```python
from build123d import *

# Parameters (mm, degrees)
EXTRUDE_1_DEPTH          = 3.5
EXTRUDE_1_DEPTH_BACK     = 3.5
SKETCH_1_R               = 2
EXTRUDE_2_DEPTH          = 7.5
EXTRUDE_2_DEPTH_BACK     = 7.5
CUT_EXTRUDE_1_DEPTH      = 2
CUT_EXTRUDE_1_DEPTH_BACK = 2
SKETCH_4_R               = 2.75
SKETCH_4_R_2             = 2
EXTRUDE_3_DEPTH          = 1.25
EXTRUDE_START            = 1.25
SKETCH_5_R               = 2.75
SKETCH_5_R_2             = 2
EXTRUDE_4_DEPTH          = 1.25
CUT_EXTRUDE_START        = -2.7500001
CUT_EXTRUDE_2_DEPTH      = 5.5000001
CUT_EXTRUDE_3_DEPTH      = 9.45
FILLET_1_R               = 0.2
FILLET_2_R               = 0.2


# Read off the part's stored shape, not the designer's step: 切除-拉伸2
with BuildPart() as part:
    # 草图1 → 凸台-拉伸1 (new, two sides: drawn at the far end of the back side and taken through both)
    with BuildSketch(Plane.XY.offset(-EXTRUDE_1_DEPTH_BACK)):
        with BuildLine():
            Line((-3.75, 7.5), (-3.75, 3.75))
            Line((-3.75, 3.75), (3.75, 3.75))
            Line((3.75, 3.75), (3.75, 7.5))
            ThreePointArc((3.75, 7.5), (0, 11.25), (-3.75, 7.5))
        make_face()
        with Locations((0, 7.5)):
            Circle(SKETCH_1_R, mode=Mode.SUBTRACT)
    extrude(amount=EXTRUDE_1_DEPTH + EXTRUDE_1_DEPTH_BACK)

    # 草图2 → 凸台-拉伸2 (add, two sides: drawn at the far end of the back side and taken through both)
    with BuildSketch(Plane.XY.offset(-EXTRUDE_2_DEPTH_BACK)):
        Polygon((-7.5, 0), (7.5, 0), (3.75, 3.75), (-3.75, 3.75), align=None)
    extrude(amount=EXTRUDE_2_DEPTH + EXTRUDE_2_DEPTH_BACK)

    # 草图3 → 切除-拉伸1 (cut, two sides: drawn at the far end of the back side and taken through both)
    with BuildSketch(Plane.XY.offset(-CUT_EXTRUDE_1_DEPTH_BACK)):
        Polygon((-2.75, 3.75), (2.75, 3.75), (2.75, 7.5), (3.75, 7.5), (3.75, 11.38728412), (-3.75, 11.38728412), (-3.75, 7.5), (-2.75, 7.5), align=None)
    extrude(amount=CUT_EXTRUDE_1_DEPTH + CUT_EXTRUDE_1_DEPTH_BACK, mode=Mode.SUBTRACT)

    # 草图4 → 凸台-拉伸3 (add)
    with BuildSketch(Plane.XY.offset(3.5)):
        with Locations((0, 7.5)):
            Circle(SKETCH_4_R)
        with Locations((0, 7.5)):
            Circle(SKETCH_4_R_2, mode=Mode.SUBTRACT)
    extrude(amount=EXTRUDE_3_DEPTH)

    # 草图5 → 凸台-拉伸4 (add)
    with BuildSketch(Plane(origin=(0, 0, -3.5), x_dir=(-1, 0, 0), z_dir=(0, 0, -1)).offset(EXTRUDE_START)):
        with Locations(Location((0, 7.5, 0), (0, 0, 180))):
            Circle(SKETCH_5_R)
        with Locations(Location((0, 7.5, 0), (0, 0, 180))):
            Circle(SKETCH_5_R_2, mode=Mode.SUBTRACT)
    extrude(amount=-EXTRUDE_4_DEPTH)

    # 切除-拉伸2 outline → 切除-拉伸2 (cut)
    with BuildSketch(Plane(origin=(0, 0, 0), x_dir=(0, 0, -1), z_dir=(1, 0, 0)).offset(CUT_EXTRUDE_START)):
        Polygon((4.75, 10.25), (3.5, 10.25), (4.75, 4.75), align=None)
        Polygon((-4.75, 10.25), (-4.75, 4.75), (-3.5, 10.25), align=None)
    extrude(amount=CUT_EXTRUDE_2_DEPTH, mode=Mode.SUBTRACT)

    # 草图7 → 切除-拉伸3 (cut)
    with BuildSketch(Plane.XY.offset(7.5)):
        with BuildLine():
            Line((-1.5, 0), (-1.5, 0.677124344))
            ThreePointArc((-1.5, 0.677124344), (-1.780042303, 1.088161527), (-1.95, 1.555590279))
            Line((-1.95, 1.555590279), (-1.95, 2.8))
            Line((-1.95, 2.8), (1.95, 2.8))
            Line((1.95, 2.8), (1.95, 1.555590279))
            ThreePointArc((1.95, 1.555590279), (1.780042303, 1.088161527), (1.5, 0.677124344))
            Line((1.5, 0.677124344), (1.5, 0))
            Line((1.5, 0), (-1.5, 0))
        make_face()
    extrude(amount=-CUT_EXTRUDE_3_DEPTH, mode=Mode.SUBTRACT)

    # 圆角1
    fillet_1_edges = [part.edges().sort_by_distance(p)[0] for p in [
        (4.5, 0, 7.5),
        (7.5, 0, 0),
        (0, 0, -7.5),
        (-7.5, 0, 0),
        (-4.5, 0, 7.5),
        (-1.5, 0, 2.775),
        (0, 0, -1.95),
        (1.5, 0, 2.775),
        (5.625, 1.875, -7.5),
        (0, 3.75, -7.5),
        (-5.625, 1.875, -7.5),
        (0, 3.75, 7.5),
        (-5.625, 1.875, 7.5),
        (5.625, 1.875, 7.5),
    ]]
    fillet(fillet_1_edges, radius=FILLET_1_R)

    # 圆角2
    fillet_2_edges = [part.edges().sort_by_distance(p)[0] for p in [
        (-3.75, 5.625, -3.5),
        (3.75, 5.625, -3.5),
        (0, 11.25, -3.5),
        (-3.75, 5.625, 3.5),
        (3.75, 5.625, 3.5),
        (0, 11.25, 3.5),
    ]]
    fillet(fillet_2_edges, radius=FILLET_2_R)


solid = part.part
```
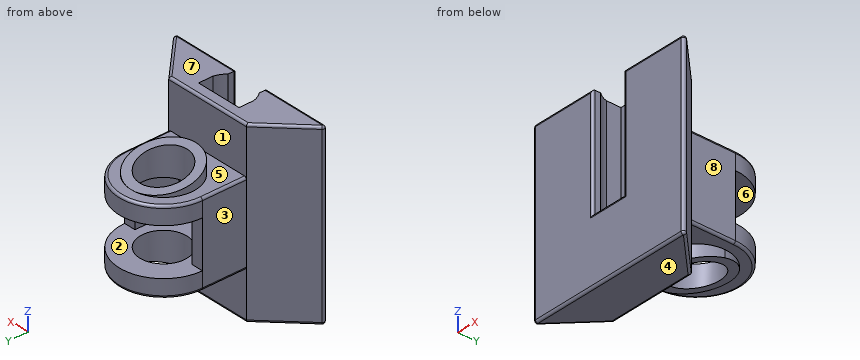
The listing builds one solid part. Answer for the finished solid, in the listing's coordinates (mm). Face numbers are marked on the shaded views. A direction names the side the tool comes from. Give positions to 0.01 mm unless a question says otherwise; leave off trailing zeros. Write each loop counter-clockwise with the first axis right and the second up, starting at its lowest first coordinate (ties: lowest second). Pieces come first, ordered by that corner, then holes. Notation, with made-up numbers: (19.25, -23) -> (37.25, -23) arc R8 cw to (37.25, -16) -> close; hole circle Ø2 at (70.5, 33). An arc over 180 degrees is marked (long way). Write item = value, one per line. Start each with the question number.
1) Which of the six approach directions +Z, -Z, +X, -X, +Y, -Y give full straight-line access (tool end or side, diameter ignored) to the marked faces 4, 5, 6, 7 and 8?
2) The part is cut by section D-D, the plane x = 1.25. Count the separate pieces of the cut face and the enclosed holes in it, and give its area (3 significant figures).
3) Determine the mould class of the marked faces 1, 2 and 3 for opening direction X: +X half, -X half, draft (parallel to the pull), parting line (faces both ways), or undercut.
4) The part is cut by section C-C, the plane z = 0.5. Determine the outline of the cut face in (x, y).
5) Straight lines are drawn through the part: line 1 along Z through (x, y) = (2, 5.25); line 2 along X through (y, z) = (7.5, 2.6); line 3 along X through (y, z) = (7.5, 3.55). For each, find the intervals that lie inside material, in ascending order.
6) Each of these flat-tipped pins is pushed along its axis until it touches: pin 1 (1 mm diameter, centred on x = -2, y = 5.5, fed in from -Z); pin 2 (2 mm diameter, centred on y = 3.5, z = 0.5, fed in from -X); pin 3 (1.9 mm diameter, centred on y = 6, z = -1, fed in from +X); pin 4 (1 mm diameter, centred on y = 8.5, z = -0.5, fed in from +X). Where does it stop, or does it pass through?
7) The part is cut by section A-A, the plane z = 2.5. Determine the outline of the cut face in (x, y).
8) The part is cut by section B-B, the plane y = 4.5. Determine the outline of the cut face in (x, z), and give its area (3 significant figures).
Solutions:
q1.face_4 = -Z, +X, -X, +Y, -Y
q1.face_5 = +Z
q1.face_6 = +Y
q1.face_7 = +Z, +X, -X, +Y, -Y
q1.face_8 = +Z, -Z, +X, +Y
q2.separate_pieces = 3
q2.enclosed_holes = 0
q2.area = 44.4 mm²
q3.face_1 = draft
q3.face_2 = undercut
q3.face_3 = -X half
q4.outline = (-7.16, 0.34) arc R0.2 ccw to (-7.02, 0) -> (-1.7, 0) arc R0.2 ccw to (-1.5, 0.2) -> (-1.5, 0.68) arc R2 cw to (-1.95, 1.56) -> (-1.95, 2.8) -> (1.95, 2.8) -> (1.95, 1.56) arc R2 cw to (1.5, 0.68) -> (1.5, 0.2) arc R0.2 ccw to (1.7, 0) -> (7.02, 0) arc R0.2 ccw to (7.16, 0.34) -> (3.75, 3.75) -> (3.75, 7.5) -> (2.75, 7.5) -> (2.75, 3.75) -> (-2.75, 3.75) -> (-2.75, 7.5) -> (-3.75, 7.5) -> (-3.75, 3.75) -> close
q5.line_1 = -3.5 to -2, 2 to 3.5
q5.line_2 = -3.75 to -2, 2 to 3.75
q5.line_3 = -2.75 to -2, 2 to 2.75
q6.pin_1 = -4.64
q6.pin_2 = -5
q6.pin_3 = 3.75
q6.pin_4 = through
q7.outline = (-7.16, 0.34) arc R0.2 ccw to (-7.02, 0) -> (-1.7, 0) arc R0.2 ccw to (-1.5, 0.2) -> (-1.5, 0.68) arc R2 cw to (-1.95, 1.56) -> (-1.95, 2.8) -> (1.95, 2.8) -> (1.95, 1.56) arc R2 cw to (1.5, 0.68) -> (1.5, 0.2) arc R0.2 ccw to (1.7, 0) -> (7.02, 0) arc R0.2 ccw to (7.16, 0.34) -> (3.75, 3.75) -> (3.75, 7.5) arc R3.75 ccw to (-3.75, 7.5) -> (-3.75, 3.75) -> close; hole circle Ø4 at (0, 7.5)
q8.outline = (-3.75, -3.3) arc R0.2 ccw to (-3.55, -3.5) -> (3.55, -3.5) arc R0.2 ccw to (3.75, -3.3) -> (3.75, 3.3) arc R0.2 ccw to (3.55, 3.5) -> (-3.55, 3.5) arc R0.2 ccw to (-3.75, 3.3) -> close; hole (-2.75, -2) -> (2.75, -2) -> (2.75, 2) -> (-2.75, 2) -> close
q8.area = 30.5 mm²
